The model under review builds one solid part; all positions refer to its coordinate system, in mm. Coordinates: 2 decimals unless noted, no trailing zeros. Write each loop counter-clockwise with the first axis right and the second up, starting at its lowest first coordinate (ties: lowest second). Pieces come first, ordered by that corner, then holes.
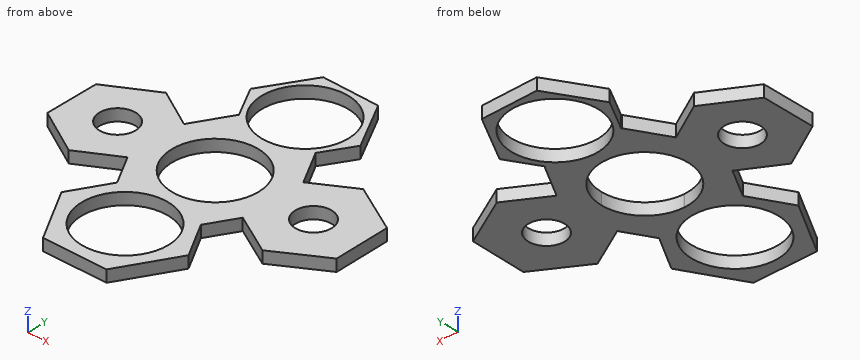
```python
from build123d import *

# Parameters (mm, degrees)
F0_R     = 11
F0_R_2   = 4.6
F1_DEPTH = 3


with BuildPart() as f1:
    # F0 (on Top) → F1 (new body)
    with BuildSketch(Plane.XY):
        with BuildLine():
            ThreePointArc((0.123785, -10.999303), (7.821817, -7.734286), (11, 0))
            ThreePointArc((11, 0), (-7.734286, 7.821817), (-0.123785, -10.999303))
            Line((-0.123785, -10.999303), (0.123785, -10.999303))
        make_face()
        with BuildLine():
            ThreePointArc((29.6, 0), (25, 4.6), (20.4, 0))
            ThreePointArc((20.4, 0), (25, -4.6), (29.6, 0))
        make_face()
        Polygon((14.973083, 8.172377), (9.939928, 17.021265), (9.727545, 17.022317), (14.377152, 24.707594), (7.503434, 37.197422), (-6.749933, 37.489521), (-14.129582, 25.291793), (-9.631268, 17.118172), (-9.770884, 17.118863), (-15.156777, 7.895989), (-24.932942, 13.604987), (-36.641381, 6.922195), (-36.708133, -6.559007), (-25.066445, -13.357416), (-15.234225, -7.745508), (-10.806813, -15.502459), (-16.290043, -24.999694), (-8.206914, -39.000084), (7.959344, -39.000084), (16.042473, -24.999694), (10.653492, -15.665704), (14.809085, -8.549611), (25.142257, -14.377539), (37.364294, -7.097444), (37.221359, 7.097444), (24.877534, 14.004538), align=None)
        with Locations((-0.123785, -24.999694)):
            Circle(F0_R, mode=Mode.SUBTRACT)
        with Locations((-24.965554, 0.140618)):
            Circle(F0_R_2, mode=Mode.SUBTRACT)
        with BuildLine():
            ThreePointArc((-0.123785, -10.999303), (-7.734286, 7.821817), (11, 0))
            ThreePointArc((11, 0), (7.821817, -7.734286), (0.123785, -10.999303))
            ThreePointArc((0.123785, -10.999303), (0, -11), (-0.123785, -10.999303))
        make_face(mode=Mode.SUBTRACT)
        with Locations((0.03405, 24.999808)):
            Circle(F0_R, mode=Mode.SUBTRACT)
        with BuildLine():
            ThreePointArc((29.6, 0), (25, -4.6), (20.4, 0))
            ThreePointArc((20.4, 0), (25, 4.6), (29.6, 0))
        make_face(mode=Mode.SUBTRACT)
    extrude(amount=F1_DEPTH)


solid = f1.part
```
Item 1: Take a section at D-D, the plane x = -28. Write out the cut boundary in (y, z), plus the area to 3 significant figures.
Solved:
outline: (-11.64, 0) - (-3.32, 0) - (-3.32, 3) - (-11.64, 3) - close; (3.6, 0) - (11.85, 0) - (11.85, 3) - (3.6, 3) - close
area: 49.8 mm2
Item 2: For pin 1 (1.5 mm diameter, centred on y = 11, z = 1, fed in from +X), flat-tipped, find the tip position at first contact; note if it passes through.
Solved:
pin 1: stops at x = 31.59
Item 3: Take a section at B-B, the plane y = 19.5. Write out the cut boundary in (x, z).
Solved:
outline: (-10.94, 0) - (-9.49, 0) - (-9.49, 3) - (-10.94, 3) - close; (9.56, 0) - (11.23, 0) - (11.23, 3) - (9.56, 3) - close
Item 4: To check wall thickness, follow line 1 along Y through (x, z) = (0, 0.8); line 2 along X through (y, z) = (-2, 0.65); line 3 along Y through (x, z) = (4, 0.8). State the ranges of each line that lie inside material, in increasing order.
Solved:
line 1: y = -39 to -36, -14 to -11, 11 to 14, 36 to 37.35
line 2: x = -36.69 to -29.04, -20.89 to -10.82, 10.82 to 20.86, 29.14 to 37.31
line 3: y = -39 to -35.2, -14.8 to -10.25, 10.25 to 14.74, 35.26 to 37.27
Item 5: Take a section at C-C, the plane x = 12. Write out the cut boundary in (y, z), plus the area to 3 significant figures.
Solved:
outline: (-32, 0) - (-18, 0) - (-18, 3) - (-32, 3) - close; (-13.36, 0) - (13.4, 0) - (13.4, 3) - (-13.36, 3) - close; (20.78, 0) - (29.03, 0) - (29.03, 3) - (20.78, 3) - close
area: 147 mm2
Item 6: Take a section at A-A, the plane x = 2. Write out the cut boundary in (y, z), plus the area to 3 significant figures.
Solved:
outline: (-39, 0) - (-35.79, 0) - (-35.79, 3) - (-39, 3) - close; (-14.21, 0) - (-10.82, 0) - (-10.82, 3) - (-14.21, 3) - close; (10.82, 0) - (14.18, 0) - (14.18, 3) - (10.82, 3) - close; (35.82, 0) - (37.31, 0) - (37.31, 3) - (35.82, 3) - close
area: 34.3 mm2
